from build123d import *

# Parameters (mm, degrees)
F1_DEPTH  = 38.1
F2_W      = 3.6068
F2_H      = 38.1
F3_DEPTH  = 6.35
F5_DEPTH  = 12.7
F6_R      = 6.35
F7_R      = 12.7
F8_W      = 6.35
F8_H      = 10.16
F9_DEPTH  = 26.9407683632
F11_DEPTH = 17.78
F13_DEPTH = 25.4


# Not quite as in the source:
# - a feature names something its author has since deleted; it is built from what else it names


with BuildPart() as f1:
    # F0 (on Top) → F1 (new body)
    with BuildSketch(Plane.XY):
        with BuildLine():
            ThreePointArc((15.4432, 0), (0, -15.4432), (-15.4432, 0))
            Line((-15.4432, 0), (-19.05, 0))
            ThreePointArc((-19.05, 0), (0, -19.05), (19.05, 0))
            Line((19.05, 0), (19.05, 39.37))
            ThreePointArc((19.05, 39.37), (17.1901280605, 43.8601280605), (12.7, 45.72))
            Line((12.7, 45.72), (-15.4432, 45.72))
            Line((-15.4432, 45.72), (-15.4432, 40.64))
            Line((-15.4432, 40.64), (6.5532, 40.64))
            Line((6.5532, 40.64), (9.0932, 40.64))
            Line((9.0932, 40.64), (15.4432, 40.64))
            Line((15.4432, 40.64), (15.4432, 34.29))
            Line((15.4432, 34.29), (15.4432, 31.75))
            Line((15.4432, 31.75), (15.4432, 0))
        make_face()
        with BuildLine():
            Line((6.5532, 40.64), (15.4432, 31.75))
            Line((15.4432, 31.75), (15.4432, 34.29))
            ThreePointArc((15.4432, 34.29), (13.5833280605, 38.7801280605), (9.0932, 40.64))
            Line((9.0932, 40.64), (6.5532, 40.64))
        make_face()
        with BuildLine():
            ThreePointArc((9.0932, 40.64), (13.5833280605, 38.7801280605), (15.4432, 34.29))
            Line((15.4432, 34.29), (15.4432, 40.64))
            Line((15.4432, 40.64), (9.0932, 40.64))
        make_face()
    extrude(amount=F1_DEPTH)

    # F2 (on Right) → F3 (join, symmetric)
    with BuildSketch(Plane.YZ):
        Polygon((-108.8525612107, 89.8025612107), (-19.05, 0), (-19.05, 38.1), (-89.8025612107, 108.8525612107), align=None)
        with Locations((-17.2466, 19.05)):
            Rectangle(F2_W, F2_H)
    extrude(amount=F3_DEPTH, both=True)

    # F4 (on face) → F5 (join, through all)
    with BuildSketch(Plane.YZ.offset(6.35)):
        Polygon((-50.3730412721, 136.93248455), (-71.8420489686, 90.8920489686), (-62.8617928475, 81.9117928475), (-41.3927851511, 127.9522284289), align=None)
    extrude(amount=-F5_DEPTH)

    # F6
    f6_edges = [f1.edges().sort_by_distance(p)[0] for p in [
        (0, -71.842049, 90.892049),
        (0, -62.861793, 81.911793),
    ]]
    fillet(f6_edges, radius=F6_R)

    # F7
    f7_edges = [f1.edges().sort_by_distance(p)[0] for p in [
        (0, -41.392785, 127.952228),
    ]]
    fillet(f7_edges, radius=F7_R)

    # F8 (on face) → F9 (join, through all)
    with BuildSketch(Plane(origin=(0, 9.525, 9.525), x_dir=(1, 0, 0), z_dir=(0, 0.7071067812, 0.7071067812))):
        with Locations((-9.525, -135.3903841816)):
            Rectangle(F8_W, F8_H)
        with Locations((9.525, -135.3903841816)):
            Rectangle(F8_W, F8_H)
        Polygon((-12.7, -130.3103841816), (-6.35, -130.3103841816), (-6.35, -124.1391240244), align=None)
        Polygon((6.35, -124.1391240244), (6.35, -130.3103841816), (12.7, -130.3103841816), align=None)
    extrude(amount=-F9_DEPTH)

    # F10 (on face) → F11 (cut)
    with BuildSketch(Plane(origin=(0, 9.525, 9.525), x_dir=(1, 0, 0), z_dir=(0, 0.7071067812, 0.7071067812))):
        Polygon((-6.35, -130.3103841816), (-3.81, -140.4703841816), (0, -140.4703841816), (0, -130.3103841816), align=None)
        Polygon((0, -130.3103841816), (0, -140.4703841816), (3.81, -140.4703841816), (6.35, -130.3103841816), align=None)
    extrude(amount=-F11_DEPTH, mode=Mode.SUBTRACT)

    # F12 (on face) → F13 (cut)
    with BuildSketch(Plane(origin=(0, 45.72, 0), x_dir=(-1, 0, 0), z_dir=(0, 1, 0))):
        with BuildLine():
            Line((-6.477, 15.3105023065), (-3.2384999613, 13.4407534373))
            ThreePointArc((-3.2384999613, 13.4407534373), (-5.6092465291, 15.8114999806), (-6.477, 19.05))
            Line((-6.477, 19.05), (-6.477, 15.3105023065))
        make_face()
        with BuildLine():
            Line((-3.2384999613, 13.4407534373), (0, 11.5710046129))
            Line((0, 11.5710046129), (0, 12.573))
            ThreePointArc((0, 12.573), (-1.6763709335, 12.7936984173), (-3.2384999613, 13.4407534373))
        make_face()
        with BuildLine():
            Line((0, 12.573), (0, 11.5710046129))
            Line((0, 11.5710046129), (3.2384995854, 13.4407532203))
            ThreePointArc((3.2384995854, 13.4407532203), (1.6763707239, 12.7936983612), (0, 12.573))
        make_face()
        with BuildLine():
            ThreePointArc((6.477, 19.05), (5.6092464206, 15.8114997927), (3.2384995854, 13.4407532203))
            Line((3.2384995854, 13.4407532203), (6.477, 15.3105023065))
            Line((6.477, 15.3105023065), (6.477, 19.05))
        make_face()
        with BuildLine():
            ThreePointArc((3.2384999681, 24.6592465587), (5.6092465311, 22.288500016), (6.477, 19.05))
            Line((6.477, 19.05), (6.477, 22.7894976935))
            Line((6.477, 22.7894976935), (3.2384999681, 24.6592465587))
        make_face()
        with BuildLine():
            Line((-6.477, 22.7894976935), (-6.477, 19.05))
            ThreePointArc((-6.477, 19.05), (-5.6092466761, 22.2884997648), (-3.2385004704, 24.6592462687))
            Line((-3.2385004704, 24.6592462687), (-6.477, 22.7894976935))
        make_face()
        with BuildLine():
            ThreePointArc((-3.2385004704, 24.6592462687), (-1.6763712174, 25.3063015066), (0, 25.527))
            Line((0, 25.527), (0, 26.5289953871))
            Line((0, 26.5289953871), (-3.2385004704, 24.6592462687))
        make_face()
        with BuildLine():
            ThreePointArc((0, 25.527), (1.6763709373, 25.3063015816), (3.2384999681, 24.6592465587))
            Line((3.2384999681, 24.6592465587), (0, 26.5289953871))
            Line((0, 26.5289953871), (0, 25.527))
        make_face()
        with BuildLine():
            Line((0, 19.05), (6.477, 19.05))
            ThreePointArc((6.477, 19.05), (5.6092465311, 22.288500016), (3.2384999681, 24.6592465587))
            ThreePointArc((3.2384999681, 24.6592465587), (1.6763709373, 25.3063015816), (0, 25.527))
            Line((0, 25.527), (0, 19.05))
        make_face()
        with BuildLine():
            Line((-6.477, 19.05), (0, 19.05))
            Line((0, 19.05), (0, 25.527))
            ThreePointArc((0, 25.527), (-1.6763712174, 25.3063015066), (-3.2385004704, 24.6592462687))
            ThreePointArc((-3.2385004704, 24.6592462687), (-5.6092466761, 22.2884997648), (-6.477, 19.05))
        make_face()
        with BuildLine():
            ThreePointArc((-3.2384999613, 13.4407534373), (-1.6763709335, 12.7936984173), (0, 12.573))
            Line((0, 12.573), (0, 19.05))
            Line((0, 19.05), (-6.477, 19.05))
            ThreePointArc((-6.477, 19.05), (-5.6092465291, 15.8114999806), (-3.2384999613, 13.4407534373))
        make_face()
        with BuildLine():
            Line((0, 19.05), (0, 12.573))
            ThreePointArc((0, 12.573), (1.6763707239, 12.7936983612), (3.2384995854, 13.4407532203))
            ThreePointArc((3.2384995854, 13.4407532203), (5.6092464206, 15.8114997927), (6.477, 19.05))
            Line((6.477, 19.05), (0, 19.05))
        make_face()
    extrude(amount=-F13_DEPTH, mode=Mode.SUBTRACT)


solid = f1.part
Can you work these out from the model? Positions are in its coordinate system, mm. A direction names the side the tool comes from. Round coordinates to 2 decimals unless told otherwise and drop trailing zeros. Order: outer loops, then holes, each group sorted by start corner. A loop starts at its lowest first (then second) coordinate and runs counter-clockwise, first axis right, second up. Notation, with made-up numbers: (19.25, 10.25) -> (50.25, 10.25) arc R28 cw to (50.25, 40.25) -> close; hole circle Ø10 at (36, 43.5). An arc over 180 degrees is marked (long way). Write each question's results on one line, items separated by ' | '. Start each with the question number.
Item 1: Will these pins go through, and if not, where does the flat tip stop? pin 1 (8 mm diameter, centred on x = -3, z = 95.5, fed in from +Y); pin 2 (5 mm diameter, centred on x = -5, y = -84, fed in from -Z); pin 3 (8 mm diameter, centred on x = 6.5, y = -57, fed in from +Z).
Item 2: If we section it at B-B, the plane y = -13: Write out the boundary of the cut face in (x, z), then the cut area to 3 significant figures.
Item 3: If we section it at D-D, the plane y = 34: Write out the boundary of the cut face in (x, z).
Item 4: If we section it at A-A, the plane x = -8.5: Write out the boundary of the cut face in (y, z).
Item 5: Thinking about a two-plate mould opening in Z: for faces 6 (the cylindrical face through (-0.09, -61.47, 82.1)), 7 (the flat face through (16, 16, 0)), 8 (the flat face through (6.35, -55, 59)), which applies, +Z half, -Z half, draft (parallel to the pull), parting line (faces both ways), or undercut?
Item 6: Which directions (+Z, -Z, +X, -X, +Y, -Y) give clear straight access to the entire face, cutting with the end or side of a thin tool? Please do faces 1 (the flat face through (0.089, -53.178, 102.679)), 2 (the cylindrical face through (0.34, -15.44, 18.78)), 3 (the flat face through (6.477, 43, 19)), 4 (the flat face through (-15.443, 43, 19)), 5 (the flat face through (10.936, 36.257, 18.783)).
Item 7: Please list where these lines run through material, in increasing order: L1, parallel to X at y = -66, z = 68; L2, parallel to Y at x = -7, z = 26; L3, parallel to Z at x = -3, y = -49.
Item 8: If we section it at C-C, the plane z = 52: Write out the boundary of the cut face in (x, y).
Results:
1) pin 1: stops at y = -54.66 | pin 2: stops at z = 62.45 | pin 3: stops at z = 131.29
2) outline: (-13.92, 0) -> (-8.34, 0) -> (-8.34, 38.1) -> (-13.92, 38.1) -> close; (8.34, 0) -> (13.92, 0) -> (13.92, 38.1) -> (8.34, 38.1) -> close | area: 426 mm2
3) outline: (13.19, 0) -> (19.05, 0) -> (19.05, 38.1) -> (13.19, 38.1) -> close
4) outline: (-108.85, 89.8) -> (-98.78, 79.73) -> (-79.73, 98.78) -> (-89.8, 108.85) -> close; (-17.05, 0) -> (-12.89, 0) -> (-12.89, 38.1) -> (-17.05, 38.1) -> close; (40.64, 0) -> (45.72, 0) -> (45.72, 38.1) -> (40.64, 38.1) -> close
5) face 6: undercut | face 7: -Z half | face 8: draft
6) face 1: +X, -X, +Y | face 2: +Z, -Z | face 3: +Y | face 4: +Z, -Z, -X, +Y | face 5: +Z, -Z, -X
7) L1: x = -6.35 to 6.35 | L2: y = -17.72 to -13.77, 40.64 to 45.72 | L3: z = 29.95 to 68.05, 111.64 to 135.56
8) outline: (-6.35, -71.05) -> (6.35, -71.05) -> (6.35, -32.95) -> (-6.35, -32.95) -> close
